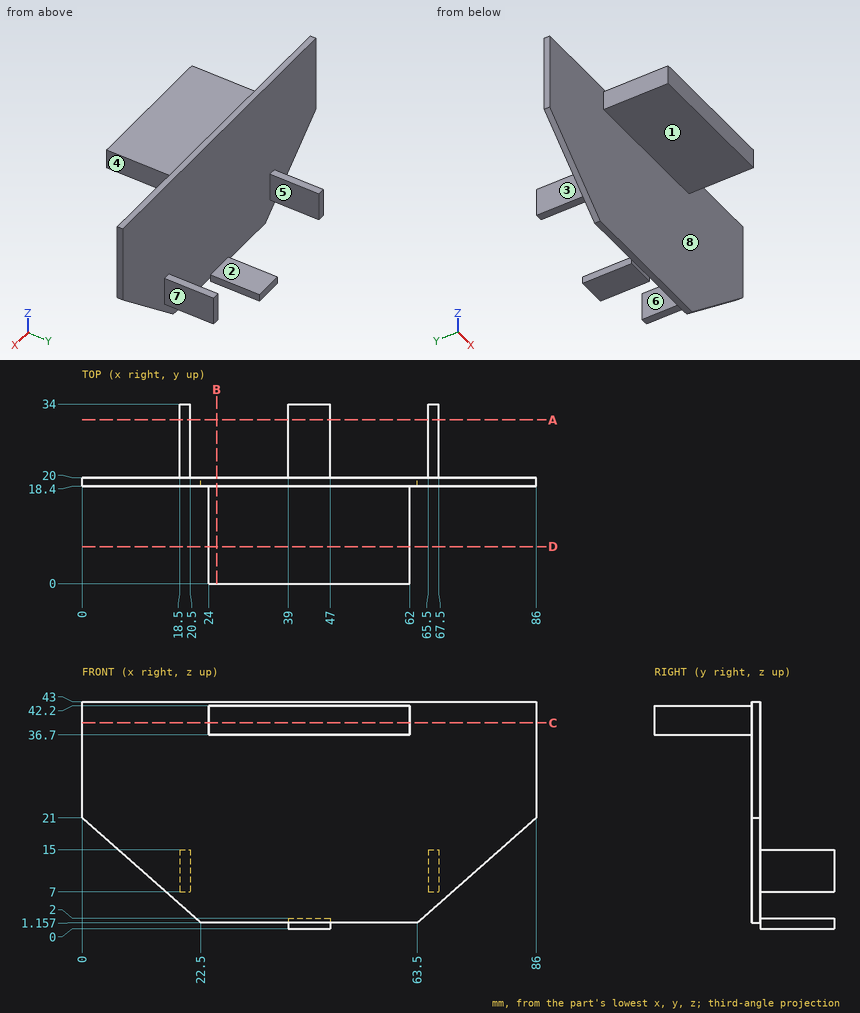
Answer from the drawing. Dimensions are ordinates in mm from the lowest x, y and z of the part. A direction names the side the tool comes from. Coordinates: 2 decimals unless noted, no trailing zeros. Write each loop counter-clockwise with the first axis right and the second up, starting at its lowest first coordinate (ties: lowest second). Pieces come first, ordered by that corner, then holes. Notation, with made-up numbers: M 10,-19.75 L 17,-19.75 A22 cw 17,8.25 Z; hole C 66,5 d4. An arc over 180 degrees is marked long. Use a Markdown table: item, result.
Q1. Which of the six approach directions +Z, -Z, +X, -X, +Y, -Y give full straight-line access (tool end or side, diameter ignored) to the marked faces 1, 2, 3 and 4?
Answer block:
| item | result |
|---|---|
| face 1 | -Z, +X, -X, -Y |
| face 2 | +Z, +X, -X, +Y |
| face 3 | +Z, -Z, -X, +Y |
| face 4 | +Z, -Z, +X, -Y |
Q2. Straight lines are drawn through the part: L1, parallel to Y at x = 63, z = 24; L2, parallel to Z at x = 60, y = 12.5; L3, parallel to Z at x = 39.5, y = 28. For each, find the intervals that lie inside material, in ascending order. Write a range as [from, to].
Answer block:
| item | result |
|---|---|
| L1 | y = [18.4, 20] |
| L2 | z = [36.7, 42.2] |
| L3 | z = [0, 2] |
Q3. The part is cut by section D-D, the plane y = 7. Write down the section's boundary in (x, z).
Answer block:
| item | result |
|---|---|
| outline | M 24,36.7 L 62,36.7 L 62,42.2 L 24,42.2 Z |
Q4. The part is cut by section B-B, the plane x = 25.5. Write down the section's boundary in (y, z).
Answer block:
| item | result |
|---|---|
| outline | M 0,36.7 L 18.4,36.7 L 18.4,1.16 L 20,1.16 L 20,43 L 18.4,43 L 18.4,42.2 L 0,42.2 Z |
Q5. Determine the mould class of the marked faces 5, 6, 7 and 8 for opening direction X: released by +X, released by -X, zero draft, split by the parting line, or undercut.
Answer block:
| item | result |
|---|---|
| face 5 | undercut |
| face 6 | undercut |
| face 7 | released by +X |
| face 8 | zero draft |
Q6. Each of these flat-tipped pins is pushed along its axis until it touches: pin 1 Ø2 at (x, y) = (66, 24.5) entering from -Z; pin 2 Ø3 at (x, z) = (42.5, 26.5) entering from +Y; pin 3 Ø0.8 at (x, y) = (36.5, 19.5) entering from -Z; pin 4 Ø3 at (y, z) = (15.5, 35) entering from +X. Where does it stop, or does it pass through?
Answer block:
| item | result |
|---|---|
| pin 1 | stops at z = 7 |
| pin 2 | stops at y = 20 |
| pin 3 | stops at z = 1.16 |
| pin 4 | passes through |
Q7. The part is cut by section C-C, the plane z = 39. Write down the section's boundary in (x, y).
Answer block:
| item | result |
|---|---|
| outline | M 0,18.4 L 24,18.4 L 24,0 L 62,0 L 62,18.4 L 86,18.4 L 86,20 L 0,20 Z |
Q8. The part is cut by section A-A, the plane y = 31. Write down the section's boundary in (x, z).
Answer block:
| item | result |
|---|---|
| outline | M 18.5,7 L 20.5,7 L 20.5,15 L 18.5,15 Z; M 39,0 L 47,0 L 47,2 L 39,2 Z; M 65.5,7 L 67.5,7 L 67.5,15 L 65.5,15 Z |
